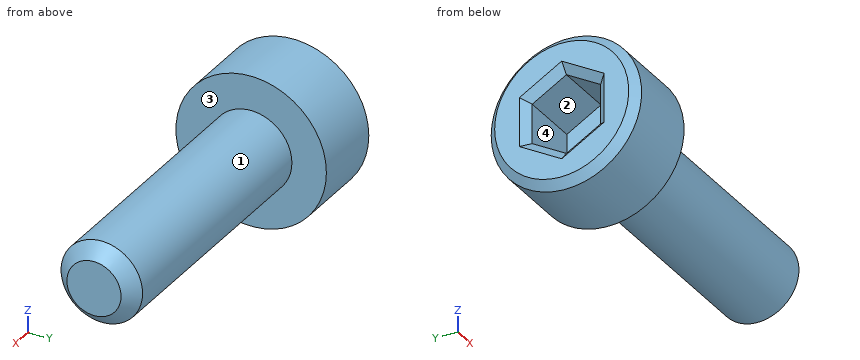
from build123d import *

# Parameters (mm, degrees)
CHAMFER1_SIZE      = 0.5
CHAMFER2_SIZE      = 0.3
CUT_EXTRUDE1_DEPTH = 2.5
CHAMFER3_SIZE      = 0.3


with BuildPart() as part:
    # Sketch1 → Revolve1 (revolve)
    with BuildSketch(Plane.XY):
        Polygon((0, 0), (0, 2.75), (3, 2.75), (3, 1.49), (13, 1.49), (13, 0), align=None)
    revolve(axis=Axis((-88.705490849, 0, 0), (1, 0, 0)))

    # Chamfer1
    chamfer1_edges = [part.edges().sort_by_distance(p)[0] for p in [
        (13, -1.49, 0),
    ]]
    chamfer(chamfer1_edges, length=CHAMFER1_SIZE)

    # Chamfer2
    chamfer2_edges = [part.edges().sort_by_distance(p)[0] for p in [
        (0, -2.75, 0),
    ]]
    chamfer(chamfer2_edges, length=CHAMFER2_SIZE)

    # Sketch3 → Cut-Extrude1 (cut)
    with BuildSketch(Plane(origin=(0, 0, 0), x_dir=(0, 0, -1), z_dir=(1, 0, 0))):
        Polygon((-1.443375673, 0), (-0.721687836, -1.25), (0.721687836, -1.25), (1.443375673, 0), (0.721687836, 1.25), (-0.721687836, 1.25), align=None)
    extrude(amount=CUT_EXTRUDE1_DEPTH, mode=Mode.SUBTRACT)

    # Chamfer3
    chamfer3_edges = [part.edges().sort_by_distance(p)[0] for p in [
        (0, 0.625, 1.082531755),
        (0, -0.625, 1.082531755),
        (0, -1.25, 0),
        (0, -0.625, -1.082531755),
        (0, 0.625, -1.082531755),
        (0, 1.25, 0),
    ]]
    chamfer(chamfer3_edges, length=CHAMFER3_SIZE)


solid = part.part
Input: part model. Units: mm. Frame: model coordinates. Face numbers are marked on the shaded views. Coordinates: 2 decimals unless noted, no trailing zeros. Loops run counter-clockwise (first coordinate to the right, second up) from the corner with the lowest first, then second, coordinate; pieces in that order, holes last.
(1) Section C-C on x = 5. Return the cut outline in (y, z).
(2) Section A-A on x = 1.5. Return the cut outline in (y, z), then the cut area to 3 significant figures.
(3) Section B-B on z = 0. Return the cut outline in (x, y), then the cut area to 3 significant figures.
(4) Pull-direction query (Y, two-part tool) for the marked faces 1, 2, 3 and 4; classes: released by +Y, released by -Y, zero draft, split by the parting line, or undercut.
(5) Material intervals for probe 1 along X at (y, z) = (1.7, -1.45); probe 2 along Y at (x, z) = (2, -0.4); probe 3 along Z at (x, y) = (2, 0.65), sorted ascending.
(6) First-contact query: pin 1 Ø1.5 at (x, z) = (10.5, -0.5) entering from +Y; pin 2 Ø1.5 at (x, y) = (4, 1.5) entering from -Z; pin 3 Ø1.5 at (x, y) = (8, 1) entering from +Z. Flat tips, straight axial feed; report the tip coordinate or a pass-through.
Data:
1. outline: circle Ø2.98 at (0, 0)
2. outline: circle Ø5.5 at (0, 0); hole (-1.25, -0.72) - (0, -1.44) - (1.25, -0.72) - (1.25, 0.72) - (0, 1.44) - (-1.25, 0.72) - close
2. area: 18.3 mm2
3. outline: (0, -2.45) - (0.3, -2.75) - (3, -2.75) - (3, -1.49) - (12.5, -1.49) - (13, -0.99) - (13, 0.99) - (12.5, 1.49) - (3, 1.49) - (3, 2.75) - (0.3, 2.75) - (0, 2.45) - (0, 1.55) - (0.3, 1.25) - (2.5, 1.25) - (2.5, -1.25) - (0.3, -1.25) - (0, -1.55) - close
3. area: 39.6 mm2
4. face 1: split by the parting line
4. face 2: undercut
4. face 3: zero draft
4. face 4: undercut
5. probe 1: x = 0 to 3
5. probe 2: y = -2.72 to -1.25, 1.25 to 2.72
5. probe 3: z = -2.67 to -1.07, 1.07 to 2.67
6. pin 1: stops at y = 1.49
6. pin 2: stops at z = -1.29
6. pin 3: stops at z = 1.47
